Read the model definition and answer for the solid it produces. Units are mm, in the model's axes. A direction names the side the tool comes from. Coordinates: 2 decimals unless noted, no trailing zeros. Write each loop counter-clockwise with the first axis right and the second up, starting at its lowest first coordinate (ties: lowest second). Pieces come first, ordered by that corner, then holes.
(1) Section C-C on y = 2.1 is taken. State how many separate pieces and enclosed holes the cut face has, then the cut area to 3 significant figures.
(2) Section B-B on z = 63 is taken. Write down the section's boundary in (x, y).
(3) The mould has two halves that part along Z. Classify faces 1 (the flat face through (-8, 3, 77)), 2 (the cylindrical face through (-5.55, 1.48, -22.83)): +Z half, -Z half, draft (parallel to the pull), parting line (faces both ways), or undercut.
(4) Given pin 1 (0.9 mm diameter, centred on y = 2, z = 109, fed in from -X); pin 2 (0.9 mm diameter, centred on y = 1.5, z = 59.5, fed in from +X), each flat-ended and moving along its own axis, determine where each tip first touches the part or whether it passes through.
(5) Find the intervals of material crossed by probe 1 along Z at (x, y) = (10, 1.3); probe 2 along X at (y, z) = (1.25, 154); probe 3 along Z at (x, y) = (14.5, 0.75), in increasing order.
(6) Which of the six approach directions +Z, -Z, +X, -X, +Y, -Y give full straight-line access (tool end or side, diameter ignored) to faces 3 (the flat face through (0.1, 1.5, 39.1)), 4 (the flat face through (-8, 0, 77))?
(7) Section A-A on z = 142 is taken. Write down the section's boundary in (x, y), then the cut area to 3 significant figures.
from build123d import *

# Parameters (mm, degrees)
SKETCH1_R           = 1.69
SKETCH1_R_2         = 1.689490446
BOSS_EXTRUDE1_DEPTH = 3


with BuildPart() as part:
    # Sketch1 → Boss-Extrude1 (new body)
    with BuildSketch(Plane(origin=(0, 0, 0), x_dir=(1, 0, 0), z_dir=(0, 1, 0))):
        Polygon((18, 28), (-18, 28), (-18, -28), (-13.5, -28), (-13.5, -128), (-18, -128), (-18, -184), (18, -184), (18, -128), (13.5, -128), (13.5, -28), (18, -28), align=None)
        with Locations(Location((-4.9, -131.61, 0), (0, 0, 270))):
            Circle(SKETCH1_R, mode=Mode.SUBTRACT)
        Polygon((-9.5, -124), (-9.5, -100.241284536), (8.065892483, -100.241284536), align=None, mode=Mode.SUBTRACT)
        Polygon((-9.5, -97.241284536), (-9.5, -84.254026063), (8.065892483, -97.241284536), align=None, mode=Mode.SUBTRACT)
        Polygon((-11, -135), (-4.9, -135), (4.9, -135), (11, -135), (11, -177), (3.865226591, -177), (2.682797031, -180.39), (-2.682797031, -180.39), (-3.865226591, -177), (-11, -177), align=None, mode=Mode.SUBTRACT)
        with Locations(Location((-4.9, -180.39, 0), (0, 0, 270))):
            Circle(SKETCH1_R, mode=Mode.SUBTRACT)
        with Locations(Location((4.9, -180.39, 0), (0, 0, 270))):
            Circle(SKETCH1_R, mode=Mode.SUBTRACT)
        with Locations(Location((4.9, -131.61, 0), (0, 0, 270))):
            Circle(SKETCH1_R, mode=Mode.SUBTRACT)
        Polygon((-5.769090987, -124), (9.5, -103.347819161), (9.5, -124), align=None, mode=Mode.SUBTRACT)
        Polygon((-8.065892483, -81.583417574), (9.5, -81.583417574), (9.5, -94.570676047), align=None, mode=Mode.SUBTRACT)
        Polygon((8.065892483, -51.718167486), (-9.5, -75.47688295), (-9.5, -51.718167486), align=None, mode=Mode.SUBTRACT)
        Polygon((-9.5, -48.718167486), (-9.5, -35.730909013), (8.065892483, -48.718167486), align=None, mode=Mode.SUBTRACT)
        Polygon((-9.5, -32), (9.5, -32), (9.5, -46.047558997), align=None, mode=Mode.SUBTRACT)
        with Locations(Location((-4.9, -24.389490446, 0), (0, 0, 270))):
            Circle(SKETCH1_R_2, mode=Mode.SUBTRACT)
        Polygon((-11, -21), (-11, 21), (-4.9, 21), (4.9, 21), (11, 21), (11, -21), (4.9, -21), align=None, mode=Mode.SUBTRACT)
        with Locations(Location((-4.9, 24.389490446, 0), (0, 0, 270))):
            Circle(SKETCH1_R_2, mode=Mode.SUBTRACT)
        Polygon((9.5, -54.82470211), (9.5, -78.583417574), (-8.065892483, -78.583417574), align=None, mode=Mode.SUBTRACT)
        with Locations(Location((4.9, -24.389490446, 0), (0, 0, 270))):
            Circle(SKETCH1_R_2, mode=Mode.SUBTRACT)
        with Locations(Location((4.9, 24.389490446, 0), (0, 0, 270))):
            Circle(SKETCH1_R_2, mode=Mode.SUBTRACT)
    extrude(amount=BOSS_EXTRUDE1_DEPTH)


solid = part.part
Response:
1. separate pieces: 1
1. enclosed holes: 18
1. area: 3,530 mm2
2. outline: (-13.5, 0) - (-9.5, 0) - (-9.5, 3) - (-13.5, 3) - close; (-0.28, 0) - (3.46, 0) - (3.46, 3) - (-0.28, 3) - close; (9.5, 0) - (13.5, 0) - (13.5, 3) - (9.5, 3) - close
3. face 1: draft
3. face 2: undercut
4. pin 1: stops at x = -13.5
4. pin 2: stops at x = 13.5
5. probe 1: z = -28 to -21, 21 to 135, 177 to 184
5. probe 2: x = -18 to -11, 11 to 18
5. probe 3: z = -28 to 28, 128 to 184
6. face 3: +Y, -Y
6. face 4: +Z, -Z, +X, -X, -Y
7. outline: (-18, 0) - (-11, 0) - (-11, 3) - (-18, 3) - close; (11, 0) - (18, 0) - (18, 3) - (11, 3) - close
7. area: 42.0 mm2
